Job drawing, mm, ordinate dimensions from the low corner. One solid piece. Give positions to 0.01 mm unless a question says otherwise; leave off trailing zeros. Order: outer loops, then holes, each group sorted by start corner. A loop starts at its lowest first (then second) coordinate and runs counter-clockwise, first axis right, second up. Notation, with made-up numbers: (10.25, -7) - (63.25, -7) arc R21 ccw to (63.25, 14) - close; hole circle Ø2 at (-20.5, 50). An arc over 180 degrees is marked (long way). One line per item, written item: value.
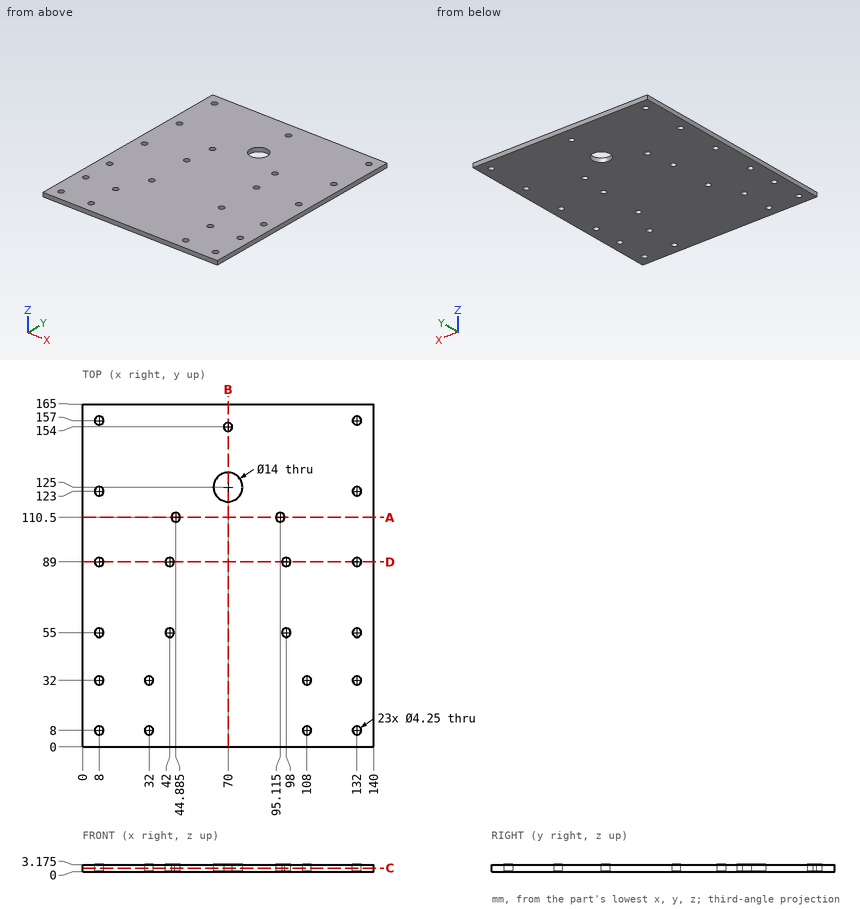
1) Slice it at A-A on y = 110.5. Write the cut outline in (x, z) (1 decimal).
Answer:
outline: (0, 0) - (42.8, 0) - (42.8, 3.2) - (0, 3.2) - close; (47, 0) - (93, 0) - (93, 3.2) - (47, 3.2) - close; (97.2, 0) - (140, 0) - (140, 3.2) - (97.2, 3.2) - close
2) Drop flat-ended pins along their axis: P1, Ø5, axis at x = 132, y = 8, coming from the +Z side (3 decimals); P2, Ø4, axis at x = 8, y = 157, coming from the +Z side. Give the stop position or say it passes through.
Answer:
P1: stops at z = 3.175
P2: passes through
3) Slice it at C-C on z = 1.7. Count the separate pieces of the cut face and the enclosed holes in it, then the cut area to 3 significant figures.
Answer:
separate pieces: 1
enclosed holes: 24
area: 22,600 mm2
4) Slice it at B-B on x = 70. Write the cut outline in (y, z) (1 decimal), then the cut area to 3 significant figures.
Answer:
outline: (0, 0) - (118, 0) - (118, 3.2) - (0, 3.2) - close; (132, 0) - (151.9, 0) - (151.9, 3.2) - (132, 3.2) - close; (156.1, 0) - (165, 0) - (165, 3.2) - (156.1, 3.2) - close
area: 466 mm2
5) Slice it at D-D on y = 89. Write the cut outline in (x, z) (1 decimal).
Answer:
outline: (0, 0) - (5.9, 0) - (5.9, 3.2) - (0, 3.2) - close; (10.1, 0) - (39.9, 0) - (39.9, 3.2) - (10.1, 3.2) - close; (44.1, 0) - (95.9, 0) - (95.9, 3.2) - (44.1, 3.2) - close; (100.1, 0) - (129.9, 0) - (129.9, 3.2) - (100.1, 3.2) - close; (134.1, 0) - (140, 0) - (140, 3.2) - (134.1, 3.2) - close
6) Wall check: line 1 along Y through (x, z) = (98, 2.3) (1 decimal); line 2 along Y through (x, z) = (71.5, 0.7) (1 decimal); line 3 along X through (y, z) = (154, 2.95) (1 decimal). Give the ranges that are in metal, low to high. Write a range as [from, to].
Answer:
line 1: y = [0, 52.9], [57.1, 86.9], [91.1, 165]
line 2: y = [0, 118.2], [131.8, 152.5], [155.5, 165]
line 3: x = [0, 67.9], [72.1, 140]
